Source: CAD feature listing. Evaluate the final solid. Frame: model axes, mm. Give positions to 0.01 mm unless a question says otherwise; leave off trailing zeros. Order: outer loops, then holes, each group sorted by start corner. A loop starts at its lowest first (then second) coordinate and runs counter-clockwise, first axis right, second up. Notation, with made-up numbers: M -2,7 L 5,7 A33 cw 5,39 Z; hole C -27.75,53 d2. An arc over 180 degrees is marked long. Answer in a Markdown table with one row per item. Add a question column.
(1) Section query A-A, the plane y = 499.5. Return loops of the section in (x, z), plus the area to 3 significant figures.
(2) Material intervals for line 1 along X through (y, z) = (194, 20.75); line 2 along Y through (x, z) = (164.5, 13); line 3 along Y through (x, z) = (916, 14.25), sorted ascending.
(3) Section query C-C, the plane x = 662. Return loops of the section in (y, z) (1 decimal), plus the area to 3 significant figures.
(4) Pin query (flat end, axial travel): P1, Ø1, axis at x = 891, z = 11, coming from the -Y side; P2, Ø1, axis at x = 681, z = 13, coming from the -Y side. Return the tip coordinate at first contact, or that it passes through.
(5) Mould query, pull axis X, two halves, no side actions, for faces 1 (the face through (1066.7, 370, 13)), 2 (the face through (0, 370, 13)), 3 (the face through (6.35, 370, 13)). Classes: pulls with the +X half, pulls with the -X half, needs draft (parallel to the pull), parting line crosses it, or undercut.
(6) Section query B-B, the plane z = 12.7. Return loops of the section in (x, y), plus the area to 3 significant figures.
from build123d import *

# Parameters (mm, degrees)
CROQUIS1_W                = 6.35
CROQUIS1_H                = 750
SALIENTE_EXTRUIR1_DEPTH   = 25.4
SALIENTE_EXTRUIR1_2_DEPTH = 25.4
CROQUIS2_R                = 4.7625
SALIENTE_EXTRUIR2_DEPTH   = 1054


with BuildPart() as part:
    # Croquis1 → Saliente-Extruir1 (new body)
    with BuildSketch(Plane.XY):
        with Locations((3.175, 375)):
            Rectangle(CROQUIS1_W, CROQUIS1_H)
    extrude(amount=SALIENTE_EXTRUIR1_DEPTH)



with BuildPart() as body_2:
    # Croquis1 → Saliente-Extruir1 2 (new body)
    with BuildSketch(Plane.XY):
        with Locations((1063.525, 375)):
            Rectangle(CROQUIS1_W, CROQUIS1_H)
    extrude(amount=SALIENTE_EXTRUIR1_2_DEPTH)


with BuildPart() as part_1:
    add(part.part)

    add(body_2.part)  # Saliente-Extruir2 merges body 2
    # Croquis2 → Saliente-Extruir2 (add)
    with BuildSketch(Plane(origin=(6.35, 0, 0), x_dir=(0, 0, -1), z_dir=(1, 0, 0))):
        with Locations(Location((-12.7, 5, 0), (0, 0, 270))):
            Circle(CROQUIS2_R)
    extrude(amount=SALIENTE_EXTRUIR2_DEPTH)


solid = part_1.part
Values follow:
| question | item | result |
|---|---|---|
| 1 | outline | M 0,0 L 6.35,0 L 6.35,25.4 L 0,25.4 Z; M 1060.35,0 L 1066.7,0 L 1066.7,25.4 L 1060.35,25.4 Z |
| 1 | area | 323 mm² |
| 2 | line 1 | x = 0 to 6.35, 1060.35 to 1066.7 |
| 2 | line 2 | y = 0.25 to 9.75 |
| 2 | line 3 | y = 0.5 to 9.5 |
| 3 | outline | C 5,12.7 d9.5 |
| 3 | area | 71.3 mm² |
| 4 | P1 | stops at y = 0.39 |
| 4 | P2 | stops at y = 0.24 |
| 5 | face 1 | pulls with the +X half |
| 5 | face 2 | pulls with the -X half |
| 5 | face 3 | undercut |
| 6 | outline | M 0,0 L 6.35,0 L 6.35,0.24 L 1060.35,0.24 L 1060.35,0 L 1066.7,0 L 1066.7,750 L 1060.35,750 L 1060.35,9.76 L 6.35,9.76 L 6.35,750 L 0,750 Z |
| 6 | area | 19,600 mm² |
